from build123d import *

# Parameters (mm, degrees)
SKETCH1_R           = 7.5
BOSS_EXTRUDE1_DEPTH = 40
SKETCH2_R           = 10
BOSS_EXTRUDE2_DEPTH = 5
CUT_EXTRUDE1_DEPTH  = 3


with BuildPart() as part:
    # Sketch1 → Boss-Extrude1 (new body)
    with BuildSketch(Plane.XY):
        Circle(SKETCH1_R)
    extrude(amount=BOSS_EXTRUDE1_DEPTH)

    # Sketch2 → Boss-Extrude2 (add)
    with BuildSketch(Plane.XY.offset(40)):
        Circle(SKETCH2_R)
    extrude(amount=BOSS_EXTRUDE2_DEPTH)

    # Sketch3 → Cut-Extrude1 (cut)
    with BuildSketch(Plane.XY.offset(45)):
        Polygon((-6.92820323, 0), (-3.464101615, -6), (3.464101615, -6), (6.92820323, 0), (3.464101615, 6), (-3.464101615, 6), align=None)
    extrude(amount=-CUT_EXTRUDE1_DEPTH, mode=Mode.SUBTRACT)


solid = part.part
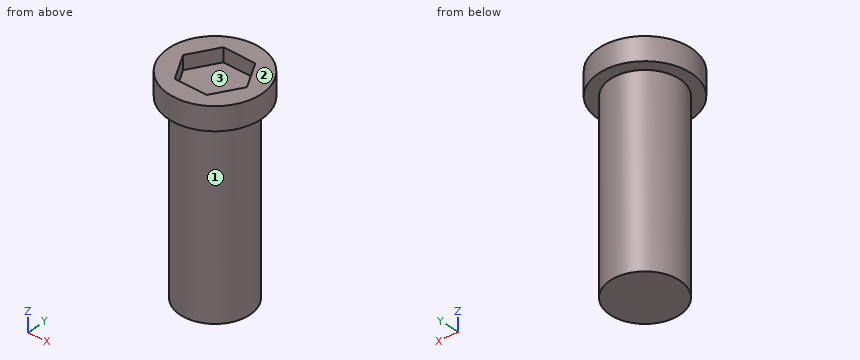
Geometry: final body of the model. Coordinates: model frame, mm. Face numbers are marked on the shaded views. Round coordinates to 2 decimals unless told otherwise and drop trailing zeros. Order: outer loops, then holes, each group sorted by start corner. A loop starts at its lowest first (then second) coordinate and runs counter-clockwise, first axis right, second up. Notation, with made-up numbers: (-26.5, -18) -> (-18.5, -18) arc R11 ccw to (-18.5, -7) -> close; hole circle Ø9 at (61.25, 10). An arc over 180 degrees is marked (long way). Put each result on its own line as item: value. Start each with the question number.
Q1. Section D-D on y = -8. Return the cut outline in (x, z), and give its area (3 significant figures).
Q2. Section C-C on z = 5.5. Return the cut outline in (x, y).
Q3. Pull-direction query (X, two-part tool) for the marked faces 1, 2 and 3; classes: +X half, -X half, draft (parallel to the pull), parting line (faces both ways), or undercut.
Q4. First-contact query: pin 1 (5 mm diameter, centred on y = -4.5, z = 10.5, fed in from -X); pin 2 (5 mm diameter, centred on y = 7, z = 36.5, fed in from -X); pin 3 (8 mm diameter, centred on y = -7, z = 18, fed in from -X). Flat tips, straight axial feed; report the tip coordinate or a pass-through.
Q5. Line query: probe 1 along Z at (x, y) = (-7, -5.75); probe 2 along Y at (x, z) = (0.25, 27); probe 3 along Z at (x, y) = (-1.5, -0.5). Output: solid intervals per line, ascending.
Q6. Section A-A on x = 0. Return the cut outline in (y, z).
Q7. Section B-B on y = 0.5. Return the cut outline in (x, z), and give its area (3 significant figures).
Ans:
1. outline: (-6, 40) -> (6, 40) -> (6, 45) -> (-6, 45) -> close
1. area: 60.0 mm2
2. outline: circle Ø15 at (0, 0)
3. face 1: parting line
3. face 2: draft
3. face 3: undercut
4. pin 1: stops at x = -7.23
4. pin 2: stops at x = -6
4. pin 3: stops at x = -6.87
5. probe 1: z = 40 to 45
5. probe 2: y = -7.5 to 7.5
5. probe 3: z = 0 to 42
6. outline: (-10, 40) -> (-7.5, 40) -> (-7.5, 0) -> (7.5, 0) -> (7.5, 40) -> (10, 40) -> (10, 45) -> (6, 45) -> (6, 42) -> (-6, 42) -> (-6, 45) -> (-10, 45) -> close
7. outline: (-9.99, 40) -> (-7.48, 40) -> (-7.48, 0) -> (7.48, 0) -> (7.48, 40) -> (9.99, 40) -> (9.99, 45) -> (6.64, 45) -> (6.64, 42) -> (-6.64, 42) -> (-6.64, 45) -> (-9.99, 45) -> close
7. area: 659 mm2
